Could you check a few things on this model? Use its own coordinates, in mm. A direction names the side the tool comes from. Give positions to 0.01 mm unless a question says otherwise; leave off trailing zeros. Write each loop counter-clockwise with the first axis right and the second up, starting at its lowest first coordinate (ties: lowest second). Pieces come first, ordered by that corner, then holes. Notation, with made-up numbers: (-11.5, 84.25) - (22.5, 84.25) arc R11 ccw to (22.5, 89.25) - close; hole circle Ø9 at (-9.75, 74). An arc over 180 degrees is marked (long way). Answer in a Markdown table with one row per item.
from build123d import *

# Parameters (mm, degrees)
SKETCH_4_R      = 5
EXTRUDE_4_DEPTH = 57
SKETCH_5_R      = 3.5
EXTRUDE_5_DEPTH = 2
EXTRUDE_START   = 10
SKETCH_6_R      = 5
EXTRUDE_6_DEPTH = 10
EXTRUDE_START_2 = 2
SKETCH_7_R      = 3.5
EXTRUDE_7_DEPTH = 2
SKETCH_8_R      = 5
EXTRUDE_8_DEPTH = 10
CHAMFER_1_SIZE  = 0.5


with BuildPart() as part:
    # 草图4 → 凸台-拉伸4 (new body)
    with BuildSketch(Plane(origin=(0, 0, 0), x_dir=(0, 0, -1), z_dir=(1, 0, 0))):
        with Locations(Location((0, 0, 0), (0, 0, 180))):
            Circle(SKETCH_4_R)
    extrude(amount=EXTRUDE_4_DEPTH)

    # 草图5 → 凸台-拉伸5 (add)
    with BuildSketch(Plane.ZY):
        Circle(SKETCH_5_R)
    extrude(amount=EXTRUDE_5_DEPTH)

    # 草图6 → 凸台-拉伸6 (add)
    with BuildSketch(Plane.ZY.offset(2).offset(EXTRUDE_START)):
        Circle(SKETCH_6_R)
    extrude(amount=-EXTRUDE_6_DEPTH)

    # 草图7 → 凸台-拉伸7 (add)
    with BuildSketch(Plane(origin=(57, 0, 0), x_dir=(0, 0, -1), z_dir=(1, 0, 0)).offset(EXTRUDE_START_2)):
        with Locations(Location((0, 0, 0), (0, 0, 180))):
            Circle(SKETCH_7_R)
    extrude(amount=-EXTRUDE_7_DEPTH)

    # 草图8 → 凸台-拉伸8 (add)
    with BuildSketch(Plane(origin=(59, 0, 0), x_dir=(0, 0, -1), z_dir=(1, 0, 0))):
        with Locations(Location((0, 0, 0), (0, 0, 180))):
            Circle(SKETCH_8_R)
    extrude(amount=EXTRUDE_8_DEPTH)

    # 倒角1
    chamfer_1_edges = [part.edges().sort_by_distance(p)[0] for p in [
        (-12, 0, -5),
        (69, 0, -5),
    ]]
    chamfer(chamfer_1_edges, length=CHAMFER_1_SIZE)


solid = part.part
1) We'd pull the mould along X, two halves only. Please class faces 1 (the face through (69, 0, 0)), 2 (the face through (-12, 0, 0)), 3 (the face through (57, 2.2, 3.3)): +X half, -X half, draft (parallel to the pull), parting line (faces both ways), or undercut.
Check values:
| item | result |
|---|---|
| face 1 | +X half |
| face 2 | -X half |
| face 3 | undercut |
2) On a 3-axis mill with a long thin cutter (end or side, diameter ignored), from which of +Z, -Z, +X, -X, +Y, -Y can I reach the whole of each face in a straight line? I mean faces 4 (the face through (64, 0, -5)), 5 (the face through (-0.986, -1.341, 3.233)). Say none if no direction works.
Check values:
| item | result |
|---|---|
| face 4 | +X, -X |
| face 5 | none |
3) Imagine slicing it at A-A (y = 0). List the corners of the cut face in (x, z) for me, then the cut area to 4 significant figures.
Check values:
| item | result |
|---|---|
| outline | (-12, -4.5) - (-11.5, -5) - (-2, -5) - (-2, -3.5) - (0, -3.5) - (0, -5) - (57, -5) - (57, -3.5) - (59, -3.5) - (59, -5) - (68.5, -5) - (69, -4.5) - (69, 4.5) - (68.5, 5) - (59, 5) - (59, 3.5) - (57, 3.5) - (57, 5) - (0, 5) - (0, 3.5) - (-2, 3.5) - (-2, 5) - (-11.5, 5) - (-12, 4.5) - close |
| area | 797.5 mm2 |
4) Imagine slicing it at C-C (x = 44). List the corners of the cut face in (y, z) for me.
Check values:
| item | result |
|---|---|
| outline | circle Ø10 at (0, 0) |
5) Will these pins go through, and if not, where does the flat tip stop? P1, Ø2, axis at x = 43.5, y = 2, coming from the +Z side; P2, Ø2, axis at x = 47.5, y = -2, coming from the -Z side; P3, Ø2, axis at x = 38.5, y = 1, coming from the -Z side; P4, Ø5, axis at x = 18, z = 3.5, coming from the +Y side.
Check values:
| item | result |
|---|---|
| P1 | stops at z = 4.9 |
| P2 | stops at z = -4.9 |
| P3 | stops at z = -5 |
| P4 | stops at y = 4.9 |
6) If I drill on line 1 (X direction, y = -2.25, z = 3); line 2 (X direction, y = -2.5, z = 4); line 3 (Z direction, x = 39, y = 0.25), over which ranges is the centre line in solid material (lowest first)?
Check values:
| item | result |
|---|---|
| line 1 | x = -12 to -2, 0 to 57, 59 to 69 |
| line 2 | x = -11.78 to -2, 0 to 57, 59 to 68.78 |
| line 3 | z = -4.99 to 4.99 |
